from build123d import *

# Parameters (mm, degrees)
F0_R     = 29.2989433696
F1_DEPTH = 99.822
F2_R     = 8.887223807
F3_DEPTH = 120.904
F5_DEPTH = 14.478
F7_DEPTH = 15.748
F8_R     = 10.6092029908
F9_DEPTH = 149.352


with BuildPart() as f1:
    # F0 (on Front) → F1 (new body)
    with BuildSketch(Plane.XZ):
        with Locations((-37.7041958272, 0)):
            Circle(F0_R)
    extrude(amount=F1_DEPTH)

    # F2 (on face) → F3 (cut)
    with BuildSketch(Plane.XZ.offset(99.822)):
        with Locations((-37.7041958272, 0)):
            Circle(F2_R)
    extrude(amount=-F3_DEPTH, mode=Mode.SUBTRACT)

    # F4 (on face) → F5 (join)
    with BuildSketch(Plane.XZ.offset(99.822)):
        with BuildLine():
            Line((-67.0031391968, 75.5516141653), (-67.0031391968, 0))
            ThreePointArc((-67.0031391968, 0), (-37.7041958272, 29.2989433696), (-8.4052524577, 0))
            Line((-8.4052524577, 0), (-8.4052524577, 75.5516141653))
            ThreePointArc((-8.4052524577, 75.5516141653), (-37.7041958272, 104.8505575349), (-67.0031391968, 75.5516141653))
        make_face()
    extrude(amount=-F5_DEPTH)

    # F6 (on face) → F7 (join)
    with BuildSketch(Plane(origin=(0, 0, 0), x_dir=(-1, 0, 0), z_dir=(0, 1, 0))):
        with BuildLine():
            Line((8.4052524577, 77.2385671735), (8.4052524577, 0))
            ThreePointArc((8.4052524577, 0), (37.7041958272, 29.2989433696), (67.0031391968, 0))
            Line((67.0031391968, 0), (67.0031391968, 77.2385671735))
            ThreePointArc((67.0031391968, 77.2385671735), (37.7041958272, 104.3438807805), (8.4052524577, 77.2385671735))
        make_face()
    extrude(amount=-F7_DEPTH)

    # F8 (on face) → F9 (cut)
    with BuildSketch(Plane(origin=(0, 0, 0), x_dir=(-1, 0, 0), z_dir=(0, 1, 0))):
        with Locations((32.7196232975, 82.2994410992)):
            Circle(F8_R)
    extrude(amount=-F9_DEPTH, mode=Mode.SUBTRACT)


solid = f1.part
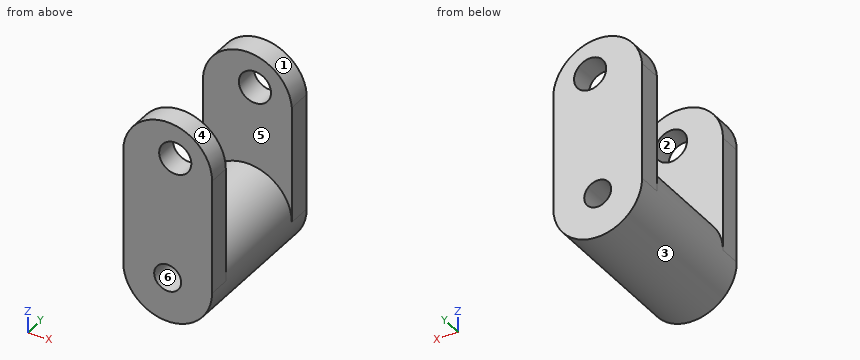
Read the model definition and answer for the solid it produces. Units are mm, in the model's axes. Face numbers are marked on the shaded views. A direction names the side the tool comes from. Round coordinates to 2 decimals unless told otherwise and drop trailing zeros. Order: outer loops, then holes, each group sorted by start corner. A loop starts at its lowest first (then second) coordinate and runs counter-clockwise, first axis right, second up.
1) The mould has two halves that part along X. Classify the marked faces 4, 5 and 6: released by +X, released by -X, zero draft, split by the parting line, or undercut.
2) The part is cut by section C-C on x = -38. Write down the section's boundary in (y, z).
3) Flat-ended cylindrical pins translate along their axes: pin 1 (10 mm diameter, centred on y = -28, z = -7, fed in from +X); pin 2 (10 mm diameter, centred on y = -46, z = 13.5, fed in from -X); pin 3 (1 mm diameter, centred on x = -27.5, y = -73.5, fed in from -Z). Find the tip coordinate at first contact, or state that the pin passes through.
4) The part is cut by section B-B on y = -22.5. Write down the section's boundary in (x, z).
5) The part is cut by section A-A on z = 50.5. Write down the section's boundary in (x, y).
6) Straight lines are drawn through the part: L1, parallel to Y at x = -43.5, z = 96; L2, parallel to X at y = -8, z = -8; L3, parallel to Z at x = -31, y = -42. For each, find the intervals that lie inside material, in ascending order.
7) The part is cut by section D-D on z = 21. Write down the section's boundary in (x, y), plus the area to 3 significant figures.
8) For the marked faces 1, 2 and 3, determine the directions among +Z, -Z, +X, -X, +Y, -Y from which every point of the face is accessible in a straight line to the end or side of a thin tool.
Resolved:
1. face 4: split by the parting line
1. face 5: zero draft
1. face 6: undercut
2. outline: (-99.82, -29.3) - (0, -29.3) - (0, -8.88) - (-99.82, -8.88) - close; (-99.82, 8.88) - (0, 8.88) - (0, 73.1) - (-15.75, 73.1) - (-15.75, 29.3) - (-85.34, 29.3) - (-85.34, 73.1) - (-99.82, 73.1) - close; (-99.82, 91.5) - (-85.34, 91.5) - (-85.34, 104.85) - (-99.82, 104.85) - close; (-15.75, 91.5) - (0, 91.5) - (0, 104.34) - (-15.75, 104.34) - close
3. pin 1: stops at x = -8.47
3. pin 2: stops at x = -65.74
3. pin 3: stops at z = -27.65
4. outline: circle Ø58.6 at (-37.7, 0); hole circle Ø17.77 at (-37.7, 0)
5. outline: (-67, -99.82) - (-8.41, -99.82) - (-8.41, -85.34) - (-67, -85.34) - close; (-67, -15.75) - (-8.41, -15.75) - (-8.41, 0) - (-67, 0) - close
6. L1: y = -99.82 to -85.34, -15.75 to 0
6. L2: x = -65.89 to -41.57, -33.83 to -9.52
6. L3: z = -28.52 to -5.83, 5.83 to 28.52
7. outline: (-67, -99.82) - (-8.41, -99.82) - (-8.41, -85.34) - (-17.27, -85.34) - (-17.27, -15.75) - (-8.41, -15.75) - (-8.41, 0) - (-67, 0) - (-67, -15.75) - (-58.14, -15.75) - (-58.14, -85.34) - (-67, -85.34) - close
7. area: 4,620 mm2
8. face 1: +Z, +Y
8. face 2: +Y, -Y
8. face 3: none
